Model file for the job. Use its own axes, mm. Coordinates: 2 decimals unless noted, no trailing zeros. Order: outer loops, then holes, each group sorted by start corner. A loop starts at its lowest first (then second) coordinate and runs counter-clockwise, first axis right, second up. Notation, with made-up numbers: M 58,79.5 L 76,79.5 A24 ccw 76,110.5 Z; hole C -29.75,-18.5 d10. An arc over 180 degrees is marked long. Return JSON: item names as keys, results as strings.
```python
from build123d import *

# Parameters (mm, degrees)
SKETCH1_R           = 2
SKETCH1_R_2         = 2.5
SKETCH1_W           = 15
SKETCH1_H           = 29
BOSS_EXTRUDE1_DEPTH = 3


with BuildPart() as part:
    # Sketch1 → Boss-Extrude1 (new body)
    with BuildSketch(Plane(origin=(0, 0, 0), x_dir=(1, 0, 0), z_dir=(0, 1, 0))):
        Polygon((-70.5, -91.713203436), (0, -21.213203436), (70.5, -91.713203436), (70.5, -109.5), (109.5, -109.5), (109.5, -70.5), (91.713203436, -70.5), (21.213203436, 0), (91.713203436, 70.5), (109.5, 70.5), (109.5, 109.5), (70.5, 109.5), (70.5, 91.713203436), (0, 21.213203436), (-70.5, 91.713203436), (-70.5, 109.5), (-109.5, 109.5), (-109.5, 70.5), (-91.713203436, 70.5), (-21.213203436, 0), (-91.713203436, -70.5), (-109.5, -70.5), (-109.5, -109.5), (-70.5, -109.5), align=None)
        with Locations((-104.5, -104.5)):
            Circle(SKETCH1_R, mode=Mode.SUBTRACT)
        with Locations((-102.5, -82.5)):
            Circle(SKETCH1_R_2, mode=Mode.SUBTRACT)
        with Locations((-77.5, -82.5)):
            Circle(SKETCH1_R_2, mode=Mode.SUBTRACT)
        with Locations((-77.5, -97.5)):
            Circle(SKETCH1_R_2, mode=Mode.SUBTRACT)
        with Locations((-102.5, -97.5)):
            Circle(SKETCH1_R_2, mode=Mode.SUBTRACT)
        with Locations((102.5, -97.5)):
            Circle(SKETCH1_R_2, mode=Mode.SUBTRACT)
        with Locations((77.5, -97.5)):
            Circle(SKETCH1_R_2, mode=Mode.SUBTRACT)
        with Locations((77.5, -82.5)):
            Circle(SKETCH1_R_2, mode=Mode.SUBTRACT)
        with Locations((102.5, -82.5)):
            Circle(SKETCH1_R_2, mode=Mode.SUBTRACT)
        with Locations((104.5, -104.5)):
            Circle(SKETCH1_R, mode=Mode.SUBTRACT)
        with Locations((104.5, 104.5)):
            Circle(SKETCH1_R, mode=Mode.SUBTRACT)
        with Locations((102.5, 82.5)):
            Circle(SKETCH1_R_2, mode=Mode.SUBTRACT)
        with Locations((77.5, 82.5)):
            Circle(SKETCH1_R_2, mode=Mode.SUBTRACT)
        with Locations((77.5, 97.5)):
            Circle(SKETCH1_R_2, mode=Mode.SUBTRACT)
        with Locations((102.5, 97.5)):
            Circle(SKETCH1_R_2, mode=Mode.SUBTRACT)
        with Locations((-102.5, 97.5)):
            Circle(SKETCH1_R_2, mode=Mode.SUBTRACT)
        with Locations((-77.5, 97.5)):
            Circle(SKETCH1_R_2, mode=Mode.SUBTRACT)
        with Locations((-77.5, 82.5)):
            Circle(SKETCH1_R_2, mode=Mode.SUBTRACT)
        with Locations((-102.5, 82.5)):
            Circle(SKETCH1_R_2, mode=Mode.SUBTRACT)
        with Locations((-104.5, 104.5)):
            Circle(SKETCH1_R, mode=Mode.SUBTRACT)
        Circle(SKETCH1_R_2, mode=Mode.SUBTRACT)
        with Locations((-10, 0)):
            Circle(SKETCH1_R_2, mode=Mode.SUBTRACT)
        with Locations((10, 0)):
            Circle(SKETCH1_R_2, mode=Mode.SUBTRACT)
        with Locations((-90, -90)):
            Rectangle(SKETCH1_W, SKETCH1_H, mode=Mode.SUBTRACT)
        with Locations((90, -90)):
            Rectangle(SKETCH1_W, SKETCH1_H, mode=Mode.SUBTRACT)
        with Locations((90, 90)):
            Rectangle(SKETCH1_W, SKETCH1_H, mode=Mode.SUBTRACT)
        with Locations((-90, 90)):
            Rectangle(SKETCH1_W, SKETCH1_H, mode=Mode.SUBTRACT)
    extrude(amount=BOSS_EXTRUDE1_DEPTH)


solid = part.part
```
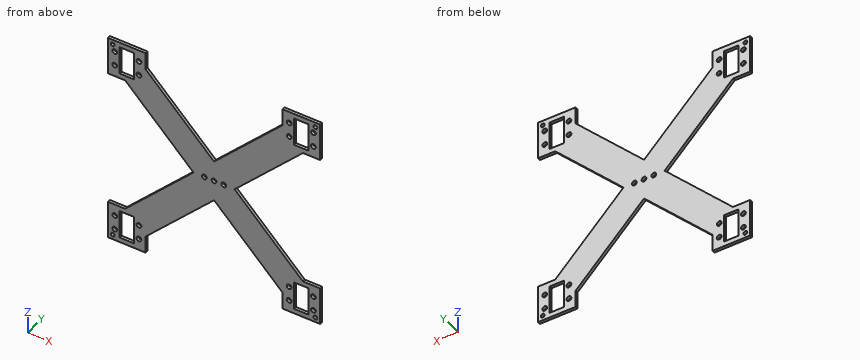
Item 1: Saw through at B-B (z = 82.5). Count the separate pieces of the cut face and the enclosed holes in it, and give its area (3 significant figures).
Check result:
{"separate pieces": "8", "enclosed holes": "0", "area": "139 mm2"}
Item 2: Saw through at D-D (x = 77.5). Write the cut outline in (y, z), and give its area (3 significant figures).
Check result:
{"outline": "M 0,-109.5 L 3,-109.5 L 3,-100 L 0,-100 Z; M 0,-95 L 3,-95 L 3,-85 L 0,-85 Z; M 0,-80 L 3,-80 L 3,-56.29 L 0,-56.29 Z; M 0,56.29 L 3,56.29 L 3,80 L 0,80 Z; M 0,85 L 3,85 L 3,95 L 0,95 Z; M 0,100 L 3,100 L 3,109.5 L 0,109.5 Z", "area": "259 mm2"}
Item 3: Drop a flat-ended pin along its axis: pin 1 Ø1.5 at (x, y) = (33, 1.5) entering from -Z. Give the stop position or say it passes through.
Check result:
{"pin 1": "stops at z = -54.96"}
Item 4: Wall check: line 1 (Z direction, x = -93, y = 1.95); line 2 (X direction, y = 1.5, z = 77); line 3 (Z direction, x = -79.5, y = 1.95). Give the ranges that are in metal, low to high.
Check result:
{"line 1": "z = -109.5 to -104.5, -75.5 to -70.5, 70.5 to 75.5, 104.5 to 109.5", "line 2": "x = -109.5 to -97.5, -82.5 to -55.79, 55.79 to 82.5, 97.5 to 109.5", "line 3": "z = -109.5 to -99, -96 to -84, -81 to -58.29, 58.29 to 81, 84 to 96, 99 to 109.5"}
Item 5: Saw through at A-A (x = 43). Write the cut outline in (y, z), and give its area (3 significant figures).
Check result:
{"outline": "M 0,-64.21 L 3,-64.21 L 3,-21.79 L 0,-21.79 Z; M 0,21.79 L 3,21.79 L 3,64.21 L 0,64.21 Z", "area": "255 mm2"}
